```python
from build123d import *

# Parameters (mm, degrees)
SKETCH2_W           = 60
SKETCH2_H           = 20
BOSS_EXTRUDE1_DEPTH = 3
SKETCH3_R           = 5
CUT_EXTRUDE1_DEPTH  = 64.316664473
SKETCH4_R           = 5
CUT_EXTRUDE2_DEPTH  = 64.316664473
FILLET1_R           = 10
FILLET2_R           = 10


with BuildPart() as part:
    # Sketch2 → Boss-Extrude1 (new body)
    with BuildSketch(Plane(origin=(0, 0, 0), x_dir=(1, 0, 0), z_dir=(0, 1, 0))):
        with Locations((30, 10)):
            Rectangle(SKETCH2_W, SKETCH2_H)
    extrude(amount=BOSS_EXTRUDE1_DEPTH)

    # Sketch3 → Cut-Extrude1 (cut, through all)
    with BuildSketch(Plane(origin=(0, 3, 0), x_dir=(1, 0, 0), z_dir=(0, 1, 0))):
        with Locations(Location((9, 10, 0), (0, 0, 270))):
            Circle(SKETCH3_R)
    extrude(amount=-CUT_EXTRUDE1_DEPTH, mode=Mode.SUBTRACT)

    # Sketch4 → Cut-Extrude2 (cut, through all)
    with BuildSketch(Plane(origin=(0, 3, 0), x_dir=(1, 0, 0), z_dir=(0, 1, 0))):
        with Locations(Location((51, 10, 0), (0, 0, 270))):
            Circle(SKETCH4_R)
    extrude(amount=-CUT_EXTRUDE2_DEPTH, mode=Mode.SUBTRACT)

    # Fillet1
    fillet1_edges = [part.edges().sort_by_distance(p)[0] for p in [
        (0, 1.5, -20),
        (0, 1.5, 0),
    ]]
    fillet(fillet1_edges, radius=FILLET1_R - 0.0001)  # a hair under: the kernel refuses the full size

    # Fillet2
    fillet2_edges = [part.edges().sort_by_distance(p)[0] for p in [
        (60, 1.5, -20),
        (60, 1.5, 0),
    ]]
    fillet(fillet2_edges, radius=FILLET2_R - 0.0001)  # a hair under: the kernel refuses the full size


solid = part.part
```
Read the model definition and answer for the solid it produces. Units are mm, in the model's axes. Give positions to 0.01 mm unless a question says otherwise; leave off trailing zeros. Order: outer loops, then holes, each group sorted by start corner. A loop starts at its lowest first (then second) coordinate and runs counter-clockwise, first axis right, second up.
(1) Find section B-B (x = 47.5). Give the vertices of the cut face in (y, z).
(2) Find section D-D (z = -10.75). Give the vertices of the cut face in (x, y).
(3) Find section A-A (y = 2.55). Give the number of separate pieces and of enclosed holes in the cut face, plus the area to 3 significant figures.
(4) Given pin 1 (1.5 mm diameter, centred on y = 2, z = -7.5, fed in from -X), flat-ended and moving along its own axis, determine where the tip first touches the part or whether it passes through.
(5) For a pull along Z with two mould halves and no side action, classify faces 1 (the flat face through (30, 0, -10)), 2 (the cylindrical face through (55, 2, -7)), 3 (the cylindrical face through (56.99, 1.52, -2.85)) as released by +Z, released by -Z, zero draft, split by the parting line, or undercut.
(6) Straight lines are drawn through the part: L1, parallel to X at y = 1.3, z = -10; L2, parallel to X at y = 2.3, z = -9; L3, parallel to Z at x = 8, y = 2.35. For each, find the intervals that lie inside material, in ascending order.
(7) Find section C-C (z = -7). Give the vertices of the cut face in (x, y).
Result sheet:
1. outline: (0, -20) - (3, -20) - (3, -13.57) - (0, -13.57) - close; (0, -6.43) - (3, -6.43) - (3, 0) - (0, 0) - close
2. outline: (0.03, 0) - (4.06, 0) - (4.06, 3) - (0.03, 3) - close; (13.94, 0) - (46.06, 0) - (46.06, 3) - (13.94, 3) - close; (55.94, 0) - (59.97, 0) - (59.97, 3) - (55.94, 3) - close
3. separate pieces: 1
3. enclosed holes: 2
3. area: 957 mm2
4. pin 1: stops at x = 0.15
5. face 1: zero draft
5. face 2: undercut
5. face 3: released by +Z
6. L1: x = 0 to 4, 14 to 46, 56 to 60
6. L2: x = 0.05 to 4.1, 13.9 to 46.1, 55.9 to 59.95
6. L3: z = -19.8 to -14.9, -5.1 to -0.2
7. outline: (0.46, 0) - (5, 0) - (5, 3) - (0.46, 3) - close; (13, 0) - (47, 0) - (47, 3) - (13, 3) - close; (55, 0) - (59.54, 0) - (59.54, 3) - (55, 3) - close
